Read the model definition and answer for the solid it produces. Units are mm, in the model's axes. Face numbers are marked on the shaded views. A direction names the side the tool comes from. Round coordinates to 2 decimals unless told otherwise and drop trailing zeros. Loops run counter-clockwise (first coordinate to the right, second up) from the corner with the lowest first, then second, coordinate; pieces in that order, holes last. Notation, with made-up numbers: (62.25, 70.5) -> (72.25, 70.5) arc R16 ccw to (72.25, 75.5) -> close; hole circle Ø3 at (42.25, 41). An arc over 180 degrees is marked (long way). Put each result on its own line as item: value.
from build123d import *

# Parameters (mm, degrees)
SKETCH1_W                       = 30
SKETCH1_H                       = 50
BOSS_EXTRUDE1_DEPTH             = 5
M4X0_7_TAPPED_HOLE1_D           = 3.3
M4X0_7_TAPPED_HOLE1_CSINK_D     = 4.55
M4X0_7_TAPPED_HOLE1_CSINK_ANGLE = 100
SKETCH4_R                       = 10
BOSS_EXTRUDE2_DEPTH             = 100
CHAMFER1_SIZE                   = 3


with BuildPart() as part:
    # Sketch1 → Boss-Extrude1 (new body)
    with BuildSketch(Plane(origin=(0, 0, 0), x_dir=(1, 0, 0), z_dir=(0, 1, 0))):
        Rectangle(SKETCH1_W, SKETCH1_H)
    extrude(amount=BOSS_EXTRUDE1_DEPTH)

    # M4x0.7 Tapped Hole1 (through all)
    with Locations(Plane(origin=(0, 5, 0), x_dir=(1, 0, 0), z_dir=(0, 1, 0))):
        with Locations((-5.5, -15), (-5.5, 0), (4.5, 0), (4.5, 15)):
            CounterSinkHole(M4X0_7_TAPPED_HOLE1_D / 2, M4X0_7_TAPPED_HOLE1_CSINK_D / 2, counter_sink_angle=M4X0_7_TAPPED_HOLE1_CSINK_ANGLE)

    # Sketch4 → Boss-Extrude2 (add)
    with BuildSketch(Plane.XZ):
        with Locations(Location((0, 0, 0), (0, 0, 90))):
            Circle(SKETCH4_R)
    extrude(amount=BOSS_EXTRUDE2_DEPTH)

    # Chamfer1
    chamfer1_edges = [part.edges().sort_by_distance(p)[0] for p in [
        (15, 2.5, 25),
        (-15, 2.5, 25),
        (-15, 2.5, -25),
        (15, 2.5, -25),
    ]]
    chamfer(chamfer1_edges, length=CHAMFER1_SIZE)


solid = part.part
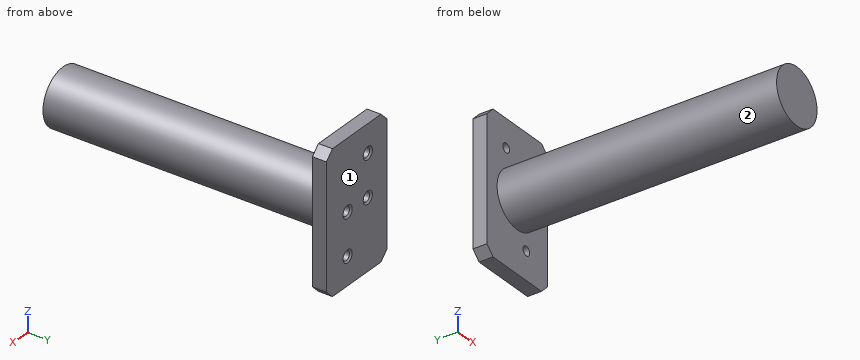
Item 1: The part is cut by section D-D (x = 8.5). Determine the outline of the cut face in (y, z).
Derived:
outline: (-100, -5.27) -> (0, -5.27) -> (0, -25) -> (5, -25) -> (5, 25) -> (0, 25) -> (0, 5.27) -> (-100, 5.27) -> close
Item 2: The part is cut by section B-B (z = 15). Determine the outline of the cut face in (x, y) (3 decimals), then the cut area to 3 significant figures.
Derived:
outline: (-15, 0) -> (-7.15, 0) -> (-7.15, 4.476) -> (-7.775, 5) -> (-15, 5) -> close; (-3.85, 0) -> (15, 0) -> (15, 5) -> (-3.225, 5) -> (-3.85, 4.476) -> close
area: 133 mm^2
Item 3: The part is cut by section A-A (x = -5.5). Determine the outline of the cut face in (y, z) (3 decimals).
Derived:
outline: (-100, -8.352) -> (0, -8.352) -> (0, -25) -> (5, -25) -> (5, -2.275) -> (4.476, -1.65) -> (0, -1.65) -> (0, 1.65) -> (4.476, 1.65) -> (5, 2.275) -> (5, 12.725) -> (4.476, 13.35) -> (0, 13.35) -> (0, 8.352) -> (-100, 8.352) -> close; (0, 16.65) -> (4.476, 16.65) -> (5, 17.275) -> (5, 25) -> (0, 25) -> close
Item 4: Which of the six approach directions +Z, -Z, +X, -X, +Y, -Y give full straight-line access (tool end or side, diameter ignored) to the marked faces 1 and 2?
Derived:
face 1: +Z, -Z, +X, -X, +Y
face 2: -Y
Item 5: The part is cut by section C-C (z = 0). Determine the outline of the cut face in (x, y) (3 decimals), then the cut area to 3 significant figures.
Derived:
outline: (-15, 0) -> (-10, 0) -> (-10, -100) -> (10, -100) -> (10, 0) -> (15, 0) -> (15, 5) -> (6.775, 5) -> (6.15, 4.476) -> (6.15, 0) -> (2.85, 0) -> (2.85, 4.476) -> (2.225, 5) -> (-3.225, 5) -> (-3.85, 4.476) -> (-3.85, 0) -> (-7.15, 0) -> (-7.15, 4.476) -> (-7.775, 5) -> (-15, 5) -> close
area: 2,120 mm^2
Item 6: Find the intervals of material crossed by line 1 along Z through (x, y) = (4.5, 3.5); line 2 along Z through (x, y) = (-5.5, 2.2); line 3 along X through (y, z) = (3, 15), in increasing order.
Derived:
line 1: z = -25 to -16.65, -13.35 to -1.65, 1.65 to 25
line 2: z = -25 to -1.65, 1.65 to 13.35, 16.65 to 25
line 3: x = -15 to -7.15, -3.85 to 15
Item 7: Flat-ended cylindrical pins translate along their axes: pin 1 Ø4 at (x, z) = (-5.5, 0) entering from +Y; pin 2 Ø2 at (x, z) = (11, -16.5) entering from -Y; pin 3 Ø2.5 at (x, z) = (-5.5, -0.5) entering from +Y. Find the tip coordinate at first contact, or state that the pin passes through.
Derived:
pin 1: stops at y = 4.77
pin 2: stops at y = 0
pin 3: stops at y = 4.56
